Part model, mm, in its own coordinate system. Face numbers are marked on the shaded views. A direction names the side the tool comes from. Coordinates: 2 decimals unless noted, no trailing zeros. Loops run counter-clockwise (first coordinate to the right, second up) from the corner with the lowest first, then second, coordinate; pieces in that order, holes last. Notation, with made-up numbers: M 39,59.25 L 51,59.25 A29 cw 51,89.25 Z; hole C 49.25,14.5 d5. An arc over 180 degrees is marked long. Answer as a JSON object with one key per item and string values. Group by question number.
1. Saw through at A-A on x = -12.25. Write the cut outline in (y, z), then the cut area to 3 significant figures.
2. Saw through at B-B on z = 317.5. Write the cut outline in (x, y), then the cut area to 3 significant figures.
3. 3-axis set-ups, long thin cutter, end or side, ignore diameter. For the marked faces 5, 6 and 7: which of +Z, -Z, +X, -X, +Y, -Y reach the whole face in a straight line?
4. Drill centre lines: L1, parallel to X at y = 375, z = 272; L2, parallel to Y at x = -12.5, z = 314.5; L3, parallel to Z at x = -14.25, y = 349.5. Where is each one in solid material? Low to high.
5. Saw through at D-D on z = 304.5. Write the cut outline in (x, y), then the cut area to 4 significant figures.
6. Saw through at C-C on y = 362. Write the cut outline in (x, z), then the cut area to 3 significant figures.
7. Mould opens along Z. For the marked faces 1, 2, 3 and 4 say: released by +Z, released by -Z, zero draft, split by the parting line, or undercut.
8. Drop flat-ended pins along their axis: pin 1 Ø1 at (x, z) = (-22.5, 278) entering from -Y; pin 2 Ø15 at (x, y) = (-16, 359) entering from -Z; pin 3 Ø4 at (x, z) = (-6.02, 258.33) entering from -Y; pin 4 Ø6 at (x, y) = (-21, 369.5) entering from +Z. Give the stop position or say it passes through.
from build123d import *

# Parameters (mm, degrees)
SKETCH1_R               = 2.15
BOSS_EXTRUDE1_DEPTH     = 5
SKETCH2_W               = 20
SKETCH2_H               = 38
BOSS_EXTRUDE2_DEPTH     = 5.5
BOSS_EXTRUDE3_START     = -5.5
SKETCH2_3_W             = 12
SKETCH2_3_H             = 5
BOSS_EXTRUDE3_DEPTH     = 1.75
BOSS_EXTRUDE4_START     = -7.25
BOSS_EXTRUDE4_DEPTH     = 12
CUT_EXTRUDE1_DEPTH      = 327.38055291
CUT_EXTRUDE1_DEPTH_BACK = 327.38055291
SKETCH3_W               = 5
SKETCH3_H               = 20
CUT_EXTRUDE2_DEPTH      = 499.511572812
CUT_EXTRUDE2_DEPTH_BACK = 499.511572812
SKETCH4_R               = 0.5


with BuildPart() as part:
    # Sketch1 → Boss-Extrude1 (new body)
    # profile 1 of 2: a face of its own
    with BuildSketch(Plane(origin=(0, 374.684836729, 0), x_dir=(1, 0, 0), z_dir=(0, 1, 0))):
        with BuildLine():
            Line((-17.462959124, -252.549454326), (-16.552371089, -253.460042361))
            ThreePointArc((-16.552371089, -253.460042361), (-5.587711318, -255.166714424), (-0.541133717, -265.049454326))
            ThreePointArc((-0.541133717, -265.049454326), (-1.047348087, -268.52729527), (-2.52398251, -271.716524237))
            ThreePointArc((-2.52398251, -271.716524237), (-2.523709833, -271.741746877), (-2.523618939, -271.766970826))
            ThreePointArc((-2.523618939, -271.766970826), (-3.566645822, -274.25961663), (-6.074066426, -275.266607243))
            ThreePointArc((-6.074066426, -275.266607243), (-20.174592051, -274.723321041), (-24.330545682, -261.238216954))
            Line((-24.330545682, -261.238216954), (-25.241133717, -260.327628919))
            Line((-25.241133717, -260.327628919), (-25.241133717, -322.549454326))
            Line((-25.241133717, -322.549454326), (-0.241133717, -322.549454326))
            Line((-0.241133717, -322.549454326), (-0.241133717, -252.549454326))
            Line((-0.241133717, -252.549454326), (-17.462959124, -252.549454326))
        make_face()
    # profile 2 of 2: a face of its own
    with BuildSketch(Plane(origin=(0, 374.684836729, 0), x_dir=(1, 0, 0), z_dir=(0, 1, 0))):
        with BuildLine():
            Line((-16.552371089, -253.460042361), (-8.852046421, -261.16036703))
            ThreePointArc((-8.852046421, -261.16036703), (-7.659796289, -262.944695448), (-7.241133717, -265.049454326))
            ThreePointArc((-7.241133717, -265.049454326), (-10.636374839, -270.130791755), (-16.630221014, -268.938541623))
            Line((-16.630221014, -268.938541623), (-24.330545682, -261.238216954))
            ThreePointArc((-24.330545682, -261.238216954), (-20.174592051, -274.723321041), (-6.074066426, -275.266607243))
            ThreePointArc((-6.074066426, -275.266607243), (-8.498492356, -269.292096775), (-2.52398251, -271.716524237))
            ThreePointArc((-2.52398251, -271.716524237), (-1.047348087, -268.52729527), (-0.541133717, -265.049454326))
            ThreePointArc((-0.541133717, -265.049454326), (-5.587711318, -255.166714424), (-16.552371089, -253.460042361))
        make_face()
        with Locations(Location((-19.458649, -271.766967887, 0), (0, 0, 270))):
            Circle(SKETCH1_R, mode=Mode.SUBTRACT)
        with Locations(Location((-6.023618435, -258.331940766, 0), (0, 0, 270))):
            Circle(SKETCH1_R, mode=Mode.SUBTRACT)
    extrude(amount=BOSS_EXTRUDE1_DEPTH)

    # Sketch2 → Boss-Extrude2 (add)
    with BuildSketch(Plane(origin=(-0.241133717, 0, 0), x_dir=(0, 0, -1), z_dir=(1, 0, 0))):
        with Locations((-312.549454326, 355.684836729)):
            Rectangle(SKETCH2_W, SKETCH2_H)
        with BuildLine():
            ThreePointArc((-308.974348052, 359.317713441), (-309.402003012, 358.785726579), (-309.54965251, 358.119319487))
            ThreePointArc((-309.54965251, 358.119319487), (-312.549454326, 355.084836729), (-315.549256143, 358.119319487))
            ThreePointArc((-315.549256143, 358.119319487), (-315.696905641, 358.785726579), (-316.124560601, 359.317713441))
            ThreePointArc((-316.124560601, 359.317713441), (-312.549454326, 369.684836729), (-308.974348052, 359.317713441))
        make_face(mode=Mode.SUBTRACT)
    extrude(amount=-BOSS_EXTRUDE2_DEPTH)

    # Sketch2<3> → Boss-Extrude3 (add)
    with BuildSketch(Plane(origin=(-0.241133717, 0, 0), x_dir=(0, 0, -1), z_dir=(1, 0, 0)).offset(BOSS_EXTRUDE3_START)):
        Polygon((-318.549454326, 374.684836729), (-322.549454326, 374.684836729), (-322.549454326, 336.684836729), (-302.549454326, 336.684836729), (-302.549454326, 374.684836729), (-306.549454326, 374.684836729), (-306.549454326, 369.684836729), (-306.549454326, 346.684836729), (-306.549454326, 341.684836729), (-318.549454326, 341.684836729), (-318.549454326, 346.684836729), (-318.549454326, 369.684836729), align=None)
        with Locations((-312.549454326, 344.184836729)):
            Rectangle(SKETCH2_3_W, SKETCH2_3_H)
        Polygon((-306.549454326, 374.684836729), (-318.549454326, 374.684836729), (-318.549454326, 369.684836729), (-312.549454326, 369.684836729), (-306.549454326, 369.684836729), align=None)
    extrude(amount=-BOSS_EXTRUDE3_DEPTH)

    # Sketch2<4> → Boss-Extrude4 (add)
    with BuildSketch(Plane(origin=(-0.241133717, 0, 0), x_dir=(0, 0, -1), z_dir=(1, 0, 0)).offset(BOSS_EXTRUDE4_START)):
        Polygon((-318.549454326, 374.684836729), (-322.549454326, 374.684836729), (-322.549454326, 336.684836729), (-302.549454326, 336.684836729), (-302.549454326, 374.684836729), (-306.549454326, 374.684836729), (-306.549454326, 369.684836729), (-306.549454326, 346.684836729), (-306.549454326, 341.684836729), (-318.549454326, 341.684836729), (-318.549454326, 346.684836729), (-318.549454326, 369.684836729), align=None)
    extrude(amount=-BOSS_EXTRUDE4_DEPTH)

    # Sketch3 → Cut-Extrude1 (cut, two sides: drawn at the far end of the back side and taken through both)
    with BuildSketch(Plane(origin=(0, 379.684836729, 0), x_dir=(1, 0, 0), z_dir=(0, 1, 0)).offset(-CUT_EXTRUDE1_DEPTH_BACK)):
        with Locations((-22.741133717, -312.549454326)):
            Rectangle(SKETCH3_W, SKETCH3_H)
    extrude(amount=CUT_EXTRUDE1_DEPTH + CUT_EXTRUDE1_DEPTH_BACK, mode=Mode.SUBTRACT)

    # Sketch4 → Cut-Extrude2 (cut, two sides: drawn at the far end of the back side and taken through both)
    with BuildSketch(Plane.ZY.offset(7.491133717).offset(-CUT_EXTRUDE2_DEPTH_BACK)):
        with Locations(Location((312.549454326, 372.184836729, 0), (0, 0, 270))):
            Circle(SKETCH4_R)
        with Locations(Location((312.549454326, 344.184836729, 0), (0, 0, 270))):
            Circle(SKETCH4_R)
    extrude(amount=CUT_EXTRUDE2_DEPTH + CUT_EXTRUDE2_DEPTH_BACK, mode=Mode.SUBTRACT)


solid = part.part
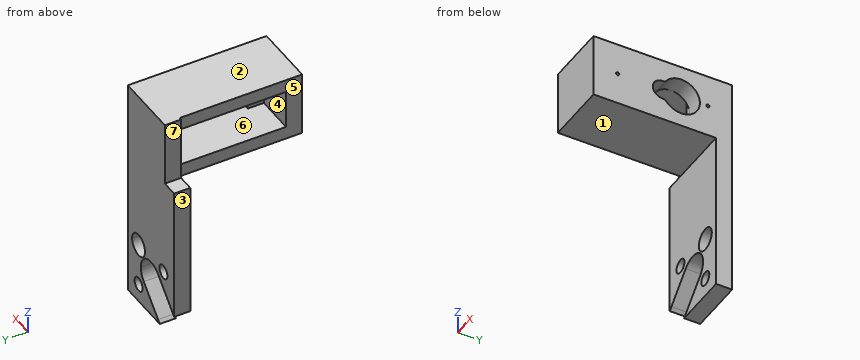
Outcome:
{
 "1": {"outline": "M 336.68,302.55 L 374.68,302.55 L 374.68,270.53 L 379.68,270.53 L 379.68,322.55 L 336.68,322.55 Z; M 374.68,252.55 L 379.68,252.55 L 379.68,257.76 L 374.68,257.76 Z; hole M 341.68,306.55 L 374.68,306.55 L 374.68,318.55 L 341.68,318.55 Z", "area": "650 mm²"},
 "2": {"outline": "M -20.24,374.68 L -7.49,374.68 L -7.49,369.68 L -5.74,369.68 L -5.74,366.91 L -0.24,366.91 L -0.24,379.68 L -20.24,379.68 Z; M -19.49,336.68 L -0.24,336.68 L -0.24,360.86 L -5.74,360.86 L -5.74,346.68 L -7.49,346.68 L -7.49,341.68 L -19.49,341.68 Z", "area": "362 mm²"},
 "3": {"face 5": "+Z, -Z, -X, -Y", "face 6": "-X", "face 7": "+Z, -X, +Y, -Y"},
 "4": {"L1": "x = -25.24 to -21.6, -17.32 to -9.52, -2.53 to -0.24", "L2": "y = 336.68 to 341.68, 374.68 to 379.68", "L3": "z = 302.55 to 306.55, 318.55 to 322.55"},
 "5": {"outline": "M -20.24,374.68 L -19.49,374.68 L -19.49,336.68 L -0.24,336.68 L -0.24,379.68 L -20.24,379.68 Z", "area": "831.5 mm²"},
 "6": {"outline": "M -19.49,302.55 L -0.24,302.55 L -0.24,307.06 L -5.74,307.06 L -5.74,306.55 L -19.49,306.55 Z; M -19.49,318.55 L -5.74,318.55 L -5.74,318.03 L -0.24,318.03 L -0.24,322.55 L -19.49,322.55 Z", "area": "160 mm²"},
 "7": {"face 1": "released by -Z", "face 2": "released by +Z", "face 3": "zero draft", "face 4": "undercut"},
 "8": {"pin 1": "stops at y = 374.68", "pin 2": "stops at z = 302.55", "pin 3": "passes through", "pin 4": "stops at z = 322.55"}
}
